Geometry: see drawing. Coordinates: mm, zero at the bounding-box minimum. A direction names the side the tool comes from. Coordinates: 2 decimals unless noted, no trailing zeros. Order: outer loops, then holes, each group sorted by start corner. A loop starts at its lowest first (then second) coordinate and runs counter-clockwise, first axis right, second up. Notation, with made-up numbers: M 83,-4.5 L 93,-4.5 A19 ccw 93,0.5 Z; hole C 64,10.5 d1. An arc over 180 degrees is marked long. One line per item, written item: value.
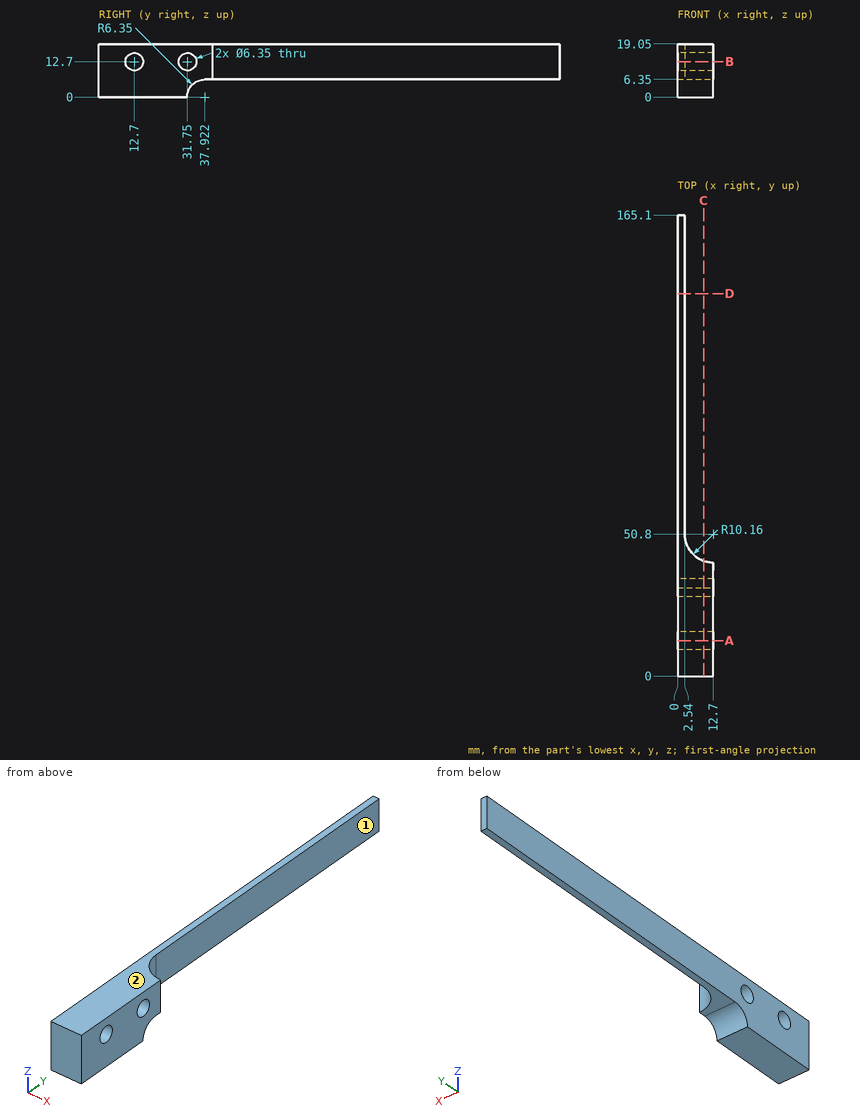
(1) Ray query, line 1 (Z direction, x = 1, y = 13); line 2 (Y direction, x = 4.5, z = 12.5); line 3 (X direction, y = 101.5, z = 6.5). Return the intervals inside material, ascending. Write a range as from..to.
Data:
line 1: z = 0..9.54, 15.86..19.05
line 2: y = 0..9.53, 15.87..28.58, 34.92..44.8
line 3: x = 0..2.54
(2) Cut plane D-D on y = 137. Output: boundary loops of the cut face in (x, z).
Data:
outline: M 0,6.35 L 2.54,6.35 L 2.54,19.05 L 0,19.05 Z
(3) Cut plane B-B on z = 12.7. Output: boundary loops of the cut face in (x, y) (3 decimals), plus the area to 3 significant figures.
Data:
outline: M 0,0 L 12.7,0 L 12.7,9.525 L 0,9.525 Z; M 0,15.875 L 12.7,15.875 L 12.7,28.575 L 0,28.575 Z; M 0,34.925 L 12.7,34.925 L 12.7,40.64 A10.16 cw 2.54,50.8 L 2.54,165.1 L 0,165.1 Z
area: 693 mm2
(4) Cut plane A-A on y = 12.7. Output: boundary loops of the cut face in (x, z) (3 decimals).
Data:
outline: M 0,0 L 12.7,0 L 12.7,9.525 L 0,9.525 Z; M 0,15.875 L 12.7,15.875 L 12.7,19.05 L 0,19.05 Z
(5) Cut plane C-C on x = 9.25. Give the number of separate pieces and of enclosed holes in the cut face, plus the area to 3 significant figures.
Data:
separate pieces: 1
enclosed holes: 2
area: 670 mm2
(6) Access query for the marked faces 1 and 2. Directions: +Z, -Z, +X, -X, +Y, -Y. A direction counts if a zero-diameter tool reaches every point of the face in a straight line with its end or side. Return the directions, or none.
Data:
face 1: +Z, -Z, +X, +Y
face 2: +Z, +X, -X, +Y, -Y
(7) First-contact query: pin 1 (1 mm diameter, centred on x = 6, z = 11.5, fed in from +Y); pin 2 (10 mm diameter, centred on y = 131.5, z = 15, fed in from +X). Flat tips, straight axial feed; report the tip coordinate or a pass-through.
Data:
pin 1: stops at y = 43.63
pin 2: stops at x = 2.54
